For this review, take the finished solid that the model builds, in its own axes (mm). Face numbers are marked on the shaded views. Coordinates: 2 decimals unless noted, no trailing zeros. Loops run counter-clockwise (first coordinate to the right, second up) from the corner with the lowest first, then second, coordinate; pieces in that order, holes last. Notation, with made-up numbers: (24, 74.25) -> (66, 74.25) arc R22 ccw to (66, 92.25) -> close; hole circle Ø10 at (3.25, -34). An arc over 180 degrees is marked (long way). Use a Markdown table: item, result.
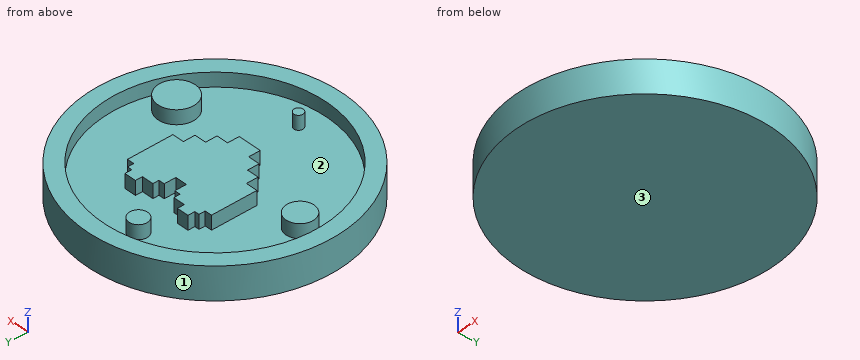
from build123d import *

# Parameters (mm, degrees)
F0_R     = 27.5
F0_R_2   = 24
F1_DEPTH = 7
F2_R     = 27.5
F3_DEPTH = 4
F4_R     = 3
F4_R_2   = 1
F4_R_3   = 4
F4_R_4   = 2
F5_DEPTH = 3
F7_DEPTH = 7


with BuildPart() as f1:
    # F0 (on Top) → F1 (new body)
    with BuildSketch(Plane.XY):
        Circle(F0_R)
        Circle(F0_R_2, mode=Mode.SUBTRACT)
    extrude(amount=F1_DEPTH)

    # F2 (on Top) → F3 (join)
    with BuildSketch(Plane.XY):
        Circle(F2_R)
    extrude(amount=F3_DEPTH)

    # F4 (on face) → F5 (join)
    with BuildSketch(Plane.XY.offset(4)):
        with Locations((-18.963763, -1.172897)):
            Circle(F4_R)
        with Locations((1.036237, -18.971721)):
            Circle(F4_R_2)
        with Locations((17.442618, -7.533598)):
            Circle(F4_R_3)
        with Locations((-2.557382, 18.827103)):
            Circle(F4_R_4)
    extrude(amount=F5_DEPTH)

    # F6 (on Top) → F7 (join)
    with BuildSketch(Plane.XY):
        Polygon((-2.5, -7.5), (0, -7.5), (2.5, -7.5), (2.5, -5), (5, -5), (5, -2.5), (7.5, -2.5), (7.5, 0), (10, 0), (10, 9.797959), (8.5, 9.797959), (8.5, 11.124298), (7.5, 11.124298), (7.5, 12.624298), (5, 12.624298), (5, 11.124298), (2.5, 11.124298), (2.5, 9.797959), (1.25, 9.797959), (1.25, 7.297959), (0, 7.297959), (-1.25, 7.297959), (-1.25, 9.797959), (-2.5, 9.797959), (-2.5, 11.124298), (-5, 11.124298), (-5, 12.624298), (-7.5, 12.624298), (-7.5, 11.124298), (-8.5, 11.124298), (-8.5, 9.797959), (-10, 9.797959), (-10, 0), (-7.5, 0), (-7.5, -2.5), (-5, -2.5), (-5, -5), (-2.5, -5), align=None)
    extrude(amount=F7_DEPTH)


solid = f1.part
(1) Take a section at A-A on z = 5.25. State how many separate pieces and enclosed holes the cut face has, plus the area to 3 significant figures.
Found:
| item | result |
|---|---|
| separate pieces | 6 |
| enclosed holes | 1 |
| area | 949 mm^2 |
(2) Take a section at B-B on x = 17. Write out the cut boundary in (y, z), plus the area to 3 significant figures.
Found:
| item | result |
|---|---|
| outline | (-21.62, 0) -> (21.62, 0) -> (21.62, 7) -> (16.94, 7) -> (16.94, 4) -> (-3.56, 4) -> (-3.56, 7) -> (-11.51, 7) -> (-11.51, 4) -> (-16.94, 4) -> (-16.94, 7) -> (-21.62, 7) -> close |
| area | 225 mm^2 |
(3) Mouldability with a two-part tool opening along Y and no side actions: class the marked faces 1, 2 and 3 as pulls with the +Y half, pulls with the -Y half, needs draft (parallel to the pull), parting line crosses it, or undercut.
Found:
| item | result |
|---|---|
| face 1 | parting line crosses it |
| face 2 | undercut |
| face 3 | needs draft |
(4) For line 1 along Y through (x, z) = (0, 5.75); line 2 along X through (y, z) = (-0.5, 5.5); line 3 along X through (y, z) = (7, 4.5), list the stretches that pass through material, from the lowest coordinate up.
Found:
| item | result |
|---|---|
| line 1 | y = -27.5 to -24, -7.5 to 7.3, 24 to 27.5 |
| line 2 | x = -27.5 to -23.99, -21.89 to -16.04, -7.5 to 7.5, 23.99 to 27.5 |
| line 3 | x = -26.59 to -22.96, -10 to 10, 22.96 to 26.59 |
(5) Take a section at C-C on y = -6.5. Write out the cut boundary in (x, z).
Found:
| item | result |
|---|---|
| outline | (-26.72, 0) -> (26.72, 0) -> (26.72, 7) -> (23.1, 7) -> (23.1, 4) -> (21.31, 4) -> (21.31, 7) -> (13.58, 7) -> (13.58, 4) -> (2.5, 4) -> (2.5, 7) -> (-2.5, 7) -> (-2.5, 4) -> (-23.1, 4) -> (-23.1, 7) -> (-26.72, 7) -> close |
(6) Take a section at D-D on y = 18. Write out the cut boundary in (x, z), plus the area to 3 significant figures.
Found:
| item | result |
|---|---|
| outline | (-20.79, 0) -> (20.79, 0) -> (20.79, 7) -> (15.87, 7) -> (15.87, 4) -> (-0.74, 4) -> (-0.74, 7) -> (-4.38, 7) -> (-4.38, 4) -> (-15.87, 4) -> (-15.87, 7) -> (-20.79, 7) -> close |
| area | 207 mm^2 |
(7) For pin 1 Ø10 at (x, y) = (21.5, -0.5) entering from -Z; pin 2 Ø3.5 at (y, z) = (5, 5) entering from -X; pin 3 Ø1.1 at (y, z) = (10.5, 5.5) entering from +X; pin 4 Ø3 at (x, z) = (4, 6) entering from -Y, all flat-tipped, find the tip position at first contact; note any pin that passes through.
Found:
| item | result |
|---|---|
| pin 1 | stops at z = 0 |
| pin 2 | stops at x = -27.31 |
| pin 3 | stops at x = 25.64 |
| pin 4 | stops at y = -27.39 |
